from build123d import *

# Parameters (mm, degrees)
SKETCH1_R              = 1
BASE_DEPTH             = 0.5
CUT_EXTRUDE6_DEPTH     = 2.5
CIRPATTERN1_COUNT      = 8
WHOLE_CONNECTION_DEPTH = 10
SKETCH1_6_R            = 0.5
ON_BEARING_DEPTH       = 5


with BuildPart() as part:
    # Sketch1 → Base (new body)
    with BuildSketch(Plane.XY):
        Circle(SKETCH1_R)
    extrude(amount=BASE_DEPTH)

    # Sketch1_3 → Cut-Extrude6 (cut, symmetric)
    with BuildSketch(Plane.XY):
        with BuildLine():
            Line((0.125, 0.75), (0.208029796, 0.978122489))
            ThreePointArc((0.208029796, 0.978122489), (0, 1), (-0.208029796, 0.978122489))
            Line((-0.208029796, 0.978122489), (-0.125, 0.75))
            Line((-0.125, 0.75), (0, 0.75))
            Line((0, 0.75), (0.125, 0.75))
        make_face()
    cut_extrude6 = extrude(amount=CUT_EXTRUDE6_DEPTH, both=True, mode=Mode.SUBTRACT)

    # CirPattern1: Cut-Extrude6 ×8 about axis
    cirpattern1_axis = Axis((0, 0, 0), (0, 0, 1))
    for i in range(1, CIRPATTERN1_COUNT):
        add(cut_extrude6.rotate(cirpattern1_axis, i * 360 / CIRPATTERN1_COUNT), mode=Mode.SUBTRACT)

    # Sketch1_5 → Whole-connection (add)
    with BuildSketch(Plane.XY):
        with BuildLine():
            Line((0.208029796, 0.454668675), (0.208029796, 0.154668675))
            Line((0.208029796, 0.154668675), (-0.208029796, 0.154668675))
            Line((-0.208029796, 0.154668675), (-0.208029796, 0.454668675))
            ThreePointArc((-0.208029796, 0.454668675), (0, -0.5), (0.208029796, 0.454668675))
        make_face()
    extrude(amount=-WHOLE_CONNECTION_DEPTH)

    # Sketch1_6 → On-bearing (add)
    with BuildSketch(Plane.XY):
        Circle(SKETCH1_6_R)
    extrude(amount=-ON_BEARING_DEPTH)


solid = part.part
For this review, take the finished solid that the model builds, in its own axes (mm). Round coordinates to 2 decimals unless told otherwise and drop trailing zeros. Write each loop counter-clockwise with the first axis right and the second up, starting at its lowest first coordinate (ties: lowest second). Pieces come first, ordered by that corner, then holes. Notation, with made-up numbers: (50.5, -7) -> (65.5, -7) arc R27 ccw to (65.5, 12) -> close; hole circle Ø11 at (-28.5, 61). An arc over 180 degrees is marked (long way). Put each result on its own line as item: value.
Q1. Consider section C-C on z = -4.5. State the section outline as (x, y) points, and give its area (3 significant figures).
Determined:
outline: circle Ø1 at (0, 0)
area: 0.785 mm^2
Q2. Consider section B-B on y = 0. State the section outline as (x, z) points, and give its area (4 significant figures).
Determined:
outline: (-0.75, 0) -> (-0.5, 0) -> (-0.5, -10) -> (0.5, -10) -> (0.5, 0) -> (0.75, 0) -> (0.75, 0.5) -> (-0.75, 0.5) -> close
area: 10.75 mm^2
Q3. To check wall thickness, follow L1, parallel to Z at x = -0.2, y = 0.7; L2, parallel to X at y = -0.05, z = -3.75; L3, parallel to Y at x = -0.05, z = -9. State the ranges of each line that lie inside material, in increasing order. Write a range as [from, to].
Determined:
L1: z = [0, 0.5]
L2: x = [-0.5, 0.5]
L3: y = [-0.5, 0.15]
Q4. Consider section D-D on z = -6.25. State the section outline as (x, y) points.
Determined:
outline: (-0.21, 0.15) -> (-0.21, 0.45) arc R0.5 ccw (long way) to (0.21, 0.45) -> (0.21, 0.15) -> close
Q5. Consider section A-A on x = 0. State the section outline as (y, z) points, and give its area (3 significant figures).
Determined:
outline: (-0.75, 0) -> (-0.5, 0) -> (-0.5, -10) -> (0.15, -10) -> (0.15, -5) -> (0.5, -5) -> (0.5, 0) -> (0.75, 0) -> (0.75, 0.5) -> (-0.75, 0.5) -> close
area: 9.02 mm^2
